Autodesk Inventor part; units mm, degrees
ref_plane "YZ Plane" through (0, 0, 0) normal (1, 0, 0) x (0, 1, 0)
ref_plane "XZ Plane" through (0, 0, 0) normal (0, 1, 0) x (-1, 0, 0)
ref_plane "XY Plane" through (0, 0, 0) normal (0, 0, 1) x (1, 0, 0)
sketch "Sketch1" plane through (0, 0, 0) normal (0, 0, 1) x (1, 0, 0)
  line L0 (707.9241, 284.5068) -> (560.717, 245.0627)
  arc A0 (560.717, 245.0627) -> (168.6533, 82.6646) centre (981.4533, -1325.1463) ccw
  line L1 (168.6533, 82.6646) -> (25.4001, -0.0426)
  line L2 (25.4001, -0.0426) -> (0.0001, 43.9515)
  line L3 (0.0001, 43.9515) -> (143.2533, 126.6587)
  arc A1 (547.569, 294.1318) -> (143.2533, 126.6587) centre (981.4533, -1325.1463) ccw
  line L4 (547.569, 294.1318) -> (694.7761, 333.5758)
  line L5 (694.7761, 333.5758) -> (707.9241, 284.5068)
  point P0 (0, 0)
extrude "Extrusion1" add sketch "Sketch1" along normal blind 19.05
properties part number "nd-o"
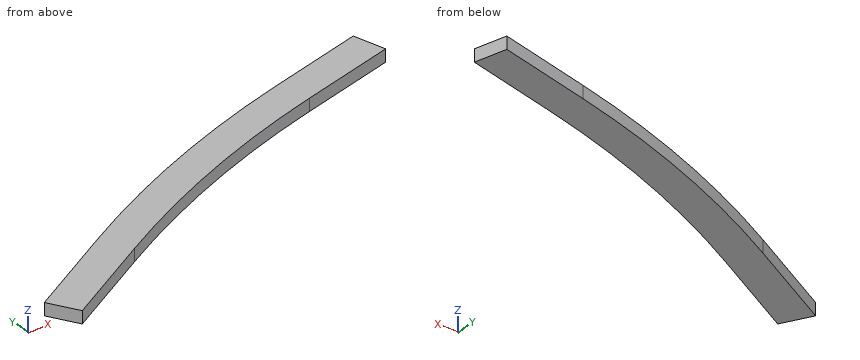
Geometry: final body of the model. Coordinates: model frame, mm. Round coordinates to 2 decimals unless told otherwise and drop trailing zeros. Loops run counter-clockwise (first coordinate to the right, second up) from the corner with the lowest first, then second, coordinate; pieces in that order, holes last. Notation, with made-up numbers: (-0.75, 20.5) -> (50.25, 20.5) arc R23 ccw to (50.25, 57.5) -> close; hole circle Ø9 at (83, -39.75). An arc over 180 degrees is marked (long way). Use one line per item in the form item = value.
Item 1: Material intervals for probe 1 along Y at (x, z) = (206.5, 2.5); probe 2 along X at (y, z) = (110, 11.25); probe 3 along X at (y, z) = (74, 8.25), sorted ascending.
Evaluation:
probe_1 = 103.85 to 161.38
probe_2 = 114.4 to 217.95
probe_3 = 52.05 to 153.65
Item 2: Contact query for flat-ended pins moving along their axis: pin 1 Ø2 at (y, z) = (120.5, 14.5) entering from +X; pin 2 Ø1 at (x, z) = (151, 4) entering from -Y; pin 3 Ø6 at (x, z) = (434, 7.5) entering from -Y. Output: stop coordinate, or through.
Evaluation:
pin_1 = 239.98
pin_2 = 72.18
pin_3 = 204.42
Item 3: Cut plane B-B on x = 282. Output: boundary loops of the cut face in (y, z), then the cut area to 3 significant figures.
Evaluation:
outline = (142.28, 0) -> (198.36, 0) -> (198.36, 19.05) -> (142.28, 19.05) -> close
area = 1,070 mm2
Item 4: Cut plane C-C on y = 137.5. Output: boundary loops of the cut face in (x, z).
Evaluation:
outline = (162.32, 0) -> (272.06, 0) -> (272.06, 19.05) -> (162.32, 19.05) -> close
Item 5: Cut plane A-A on z = 4.5. Output: boundary loops of the cut face in (x, y).
Evaluation:
outline = (0, 43.95) -> (25.4, -0.04) -> (168.65, 82.66) arc R1625.6 cw to (560.72, 245.06) -> (707.92, 284.51) -> (694.78, 333.58) -> (547.57, 294.13) arc R1676.4 ccw to (143.25, 126.66) -> close
